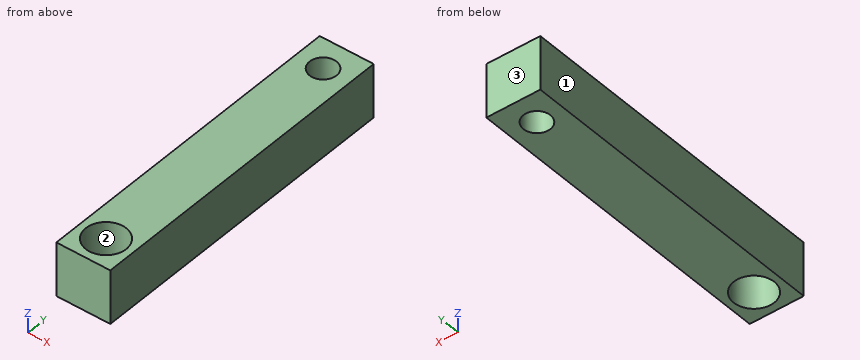
from build123d import *

# Parameters (mm, degrees)
F0_W     = 20
F0_H     = 120
F1_DEPTH = 20
F4_D     = 15
F6_D     = 10


with BuildPart() as f1:
    # F0 (on Top) → F1 (new body)
    with BuildSketch(Plane.XY):
        Rectangle(F0_W, F0_H)
    extrude(amount=F1_DEPTH)

    # F4 (through all)
    with Locations(Plane.XY.offset(20)):
        with Locations((0, -49.655378)):
            Hole(F4_D / 2)

    # F6 (through all)
    with Locations(Plane.XY.offset(20)):
        with Locations((0, 49.241364)):
            Hole(F6_D / 2)


solid = f1.part
Part model, mm, in its own coordinate system. Face numbers are marked on the shaded views. Give positions to 0.01 mm unless a question says otherwise; leave off trailing zeros. Write each loop counter-clockwise with the first axis right and the second up, starting at its lowest first coordinate (ties: lowest second). Pieces come first, ordered by that corner, then holes.
1) Pin check, flat tip, straight feed: pin 1 (9 mm diameter, centred on x = 0, y = -49.66, fed in from +Z). Stop position of the tip, or through.
Resolved:
pin 1: passes through
2) Cut at B-B on x = -6.25. Write the cut outline in (y, z).
Resolved:
outline: (-60, 0) - (-53.8, 0) - (-53.8, 20) - (-60, 20) - close; (-45.51, 0) - (60, 0) - (60, 20) - (-45.51, 20) - close
3) Cut at C-C on z = 13. Write the cut outline in (x, y).
Resolved:
outline: (-10, -60) - (10, -60) - (10, 60) - (-10, 60) - close; hole circle Ø15 at (0, -49.66); hole circle Ø10 at (0, 49.24)
4) Probe L1, parallel to Y at x = 0, z = 4.5; L2, parallel to Y at x = -2.5, z = 14.25; L3, parallel to Y at x = 6, z = 12.25. List the from-to ranges inside material, lowest first.
Resolved:
L1: y = -60 to -57.16, -42.16 to 44.24, 54.24 to 60
L2: y = -60 to -56.73, -42.58 to 44.91, 53.57 to 60
L3: y = -60 to -54.16, -45.16 to 60
5) Two-plate mould, pull along X, no slides. Class the marked faces 1, 2 and 3: released by +X, released by -X, zero draft, split by the parting line, or undercut.
Resolved:
face 1: released by -X
face 2: undercut
face 3: zero draft
6) Cut at A-A on x = 0. Write the cut outline in (y, z), then the cut area to 3 significant figures.
Resolved:
outline: (-60, 0) - (-57.16, 0) - (-57.16, 20) - (-60, 20) - close; (-42.16, 0) - (44.24, 0) - (44.24, 20) - (-42.16, 20) - close; (54.24, 0) - (60, 0) - (60, 20) - (54.24, 20) - close
area: 1,900 mm2
